```python
from build123d import *

# Parameters (mm, degrees)
SKETCH1_W           = 116
SKETCH1_H           = 79
SKETCH1_W_2         = 112
SKETCH1_H_2         = 75
BOSS_EXTRUDE1_DEPTH = 28
SKETCH2_W           = 116
SKETCH2_H           = 79
BOSS_EXTRUDE2_DEPTH = 2
SKETCH3_W           = 73
SKETCH3_H           = 48
CUT_EXTRUDE1_DEPTH  = 2
SKETCH4_R           = 1.75
CUT_EXTRUDE2_DEPTH  = 2


with BuildPart() as part:
    # Sketch1 → Boss-Extrude1 (new body)
    with BuildSketch(Plane(origin=(0, 0, 0), x_dir=(1, 0, 0), z_dir=(0, 1, 0))):
        Rectangle(SKETCH1_W, SKETCH1_H)
        Rectangle(SKETCH1_W_2, SKETCH1_H_2, mode=Mode.SUBTRACT)
    extrude(amount=BOSS_EXTRUDE1_DEPTH)

    # Sketch2 → Boss-Extrude2 (add)
    with BuildSketch(Plane(origin=(0, 28, 0), x_dir=(1, 0, 0), z_dir=(0, 1, 0))):
        Rectangle(SKETCH2_W, SKETCH2_H)
    extrude(amount=BOSS_EXTRUDE2_DEPTH)

    # Sketch3 → Cut-Extrude1 (cut)
    with BuildSketch(Plane(origin=(0, 30, 0), x_dir=(1, 0, 0), z_dir=(0, 1, 0))):
        Rectangle(SKETCH3_W, SKETCH3_H)
    extrude(amount=-CUT_EXTRUDE1_DEPTH, mode=Mode.SUBTRACT)

    # Sketch4 → Cut-Extrude2 (cut)
    with BuildSketch(Plane(origin=(0, 30, 0), x_dir=(1, 0, 0), z_dir=(0, 1, 0))):
        with Locations((50, -27.5)):
            Circle(SKETCH4_R)
    extrude(amount=-CUT_EXTRUDE2_DEPTH, mode=Mode.SUBTRACT)


solid = part.part
```
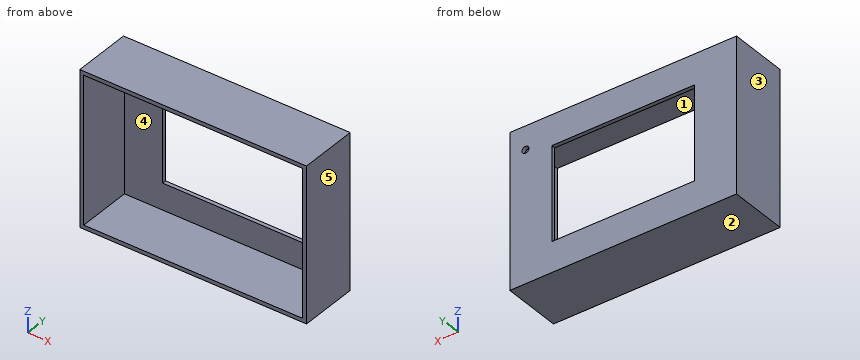
Can you work these out from the model? Positions are in its coordinate system, mm. Face numbers are marked on the shaded views. A direction names the side the tool comes from. Give positions to 0.01 mm unless a question says otherwise; leave off trailing zeros. Loops run counter-clockwise (first coordinate to the right, second up) from the corner with the lowest first, then second, coordinate; pieces in that order, holes last. Notation, with made-up numbers: M 87,19 L 100,19 A12 ccw 100,24 Z; hole C 20.5,-36.75 d4. An arc over 180 degrees is marked long. One line per item, written item: value.
(1) I need wall thicknesses on line 1 (X direction, y = 29.4, z = 27.5); line 2 (Z direction, x = -26.5, y = 21.25); line 3 (Z direction, x = 50, y = 28.55). Which ranges of each line are inside material? Lowest first, please.
Returned:
line 1: -58 to 48.25, 51.75 to 58
line 2: -39.5 to -37.5, 37.5 to 39.5
line 3: -39.5 to 25.75, 29.25 to 39.5
(2) Suppose I cut it at A-A on x = 50. List the corners of the cut face in (y, z) for me.
Returned:
outline: M 0,-39.5 L 30,-39.5 L 30,25.75 L 28,25.75 L 28,-37.5 L 0,-37.5 Z; M 0,37.5 L 28,37.5 L 28,29.25 L 30,29.25 L 30,39.5 L 0,39.5 Z
(3) Which directions (+Z, -Z, +X, -X, +Y, -Y) give clear straight access to the entire face, cutting with the end or side of a thin tool? Please do the marked faces 1 and 2.
Returned:
face 1: -Y
face 2: -Z, +X, -X, +Y, -Y
(4) Suppose I cut it at D-D on x = -47.5. List the corners of the cut face in (y, z) for me.
Returned:
outline: M 0,-39.5 L 30,-39.5 L 30,39.5 L 0,39.5 L 0,37.5 L 28,37.5 L 28,-37.5 L 0,-37.5 Z
(5) Will this pin go through, and if not, where does the flat tip stop? pin 1 (8 mm diameter, centred on x = -45, z = 5.5, fed in from -Y).
Returned:
pin 1: y = 28
(6) We'd pull the mould along X, two halves only. Please class the marked faces 3, 4 and 5: released by +X, released by -X, zero draft, split by the parting line, or undercut.
Returned:
face 3: released by -X
face 4: undercut
face 5: released by +X
(7) Suppose I cut it at B-B on z = 27.5. List the corners of the cut face in (x, y) for me, plus the area to 3 significant figures.
Returned:
outline: M -58,0 L -56,0 L -56,28 L 48.25,28 L 48.25,30 L -58,30 Z; M 51.75,28 L 56,28 L 56,0 L 58,0 L 58,30 L 51.75,30 Z
area: 337 mm^2
(8) Suppose I cut it at C-C on y = 25.25. List the corners of the cut face in (x, z) for me.
Returned:
outline: M -58,-39.5 L 58,-39.5 L 58,39.5 L -58,39.5 Z; hole M -56,-37.5 L 56,-37.5 L 56,37.5 L -56,37.5 Z
